Read the model definition and answer for the solid it produces. Units are mm, in the model's axes. Face numbers are marked on the shaded views. A direction names the side the tool comes from. Coordinates: 2 decimals unless noted, no trailing zeros. Write each loop counter-clockwise with the first axis right and the second up, starting at its lowest first coordinate (ties: lowest second). Pieces come first, ordered by that corner, then holes.
from build123d import *

# Parameters (mm, degrees)
BOSS_EXTRUDE1_DEPTH      = 50
BOSS_EXTRUDE1_DEPTH_BACK = 50
SKETCH1_W                = 180
SKETCH1_H                = 152.061
SHELL1_T                 = -5
SKETCH3_W                = 170
SKETCH3_H                = 142.061
BOSS_EXTRUDE2_DEPTH      = 37
CUT_EXTRUDE1_REACH       = 203.694
SKETCH2_W                = 36
SKETCH2_H                = 58
SKETCH4_W                = 36
SKETCH4_H                = 46.5
SKETCH4_R                = 1.5
CUT_EXTRUDE2_DEPTH       = 2
SKETCH4_3_R              = 1.5
CUT_EXTRUDE3_DEPTH       = 132.318836921
SKETCH5_W                = 159.952904784
SKETCH5_H                = 5
CUT_EXTRUDE4_DEPTH       = 63
SKETCH8_W                = 72
SKETCH8_H                = 29.937457508
CUT_EXTRUDE5_DEPTH       = 37
SKETCH9_R                = 1.5
CUT_EXTRUDE6_DEPTH       = 10
CUT_EXTRUDE7_DEPTH       = 102
FILLET1_R                = 10
SKETCH11_W               = 62
SKETCH11_H               = 5
BOSS_EXTRUDE3_DEPTH      = 100
SKETCH12_W               = 57
SKETCH12_H               = 3
SKETCH12_W_2             = 43
SKETCH12_H_2             = 2
CUT_EXTRUDE8_DEPTH       = 91
SKETCH13_W               = 57
SKETCH13_H               = 3
CUT_EXTRUDE9_DEPTH       = 7
FILLET2_R                = 10
FILLET3_R                = 100
SKETCH15_R               = 4
CUT_EXTRUDE10_DEPTH      = 28


with BuildPart() as part:
    # Sketch1 → Boss-Extrude1 (new, two sides: drawn at the far end of the back side and taken through both)
    with BuildSketch(Plane(origin=(0, 0, 0), x_dir=(1, 0, 0), z_dir=(0, 1, 0)).offset(-BOSS_EXTRUDE1_DEPTH_BACK)):
        Rectangle(SKETCH1_W, SKETCH1_H)
    extrude(amount=BOSS_EXTRUDE1_DEPTH + BOSS_EXTRUDE1_DEPTH_BACK)

    # Shell1
    shell1_openings = [part.faces().sort_by_distance(p)[0] for p in [
        (0, -50, 0),
    ]]
    offset(amount=SHELL1_T, openings=shell1_openings, kind=Kind.INTERSECTION)

    # Sketch3 → Boss-Extrude2 (add)
    with BuildSketch(Plane.XZ.offset(-45)):
        Rectangle(SKETCH3_W, SKETCH3_H)
    extrude(amount=BOSS_EXTRUDE2_DEPTH)

    # Sketch2 → Cut-Extrude1 (cut, up to next)
    with BuildSketch(Plane.ZY.offset(90), mode=Mode.PRIVATE) as cut_extrude1_sk1:
        with Locations((-46.0305, -21)):
            Rectangle(SKETCH2_W, SKETCH2_H)
    cut_extrude1_tool1 = extrude(cut_extrude1_sk1.sketch, amount=-CUT_EXTRUDE1_REACH, mode=Mode.PRIVATE) & part.part
    cut_extrude1 = cut_extrude1_tool1.solids().sort_by_distance((-90, -21, -46.0305))[0]
    add(cut_extrude1, mode=Mode.SUBTRACT)

    # Mirror1: Cut-Extrude1 across plane
    add(cut_extrude1.mirror(Plane(origin=(0, 0, 0), x_dir=(0, 0, 1), z_dir=(1, 0, 0))), mode=Mode.SUBTRACT)

    # Sketch4 → Cut-Extrude2 (cut)
    with BuildSketch(Plane.XZ.offset(-8)):
        with Locations((-54, -34.0305)):
            Rectangle(SKETCH4_W, SKETCH4_H)
        with Locations(Location((-43, -50.2805, 0), (0, 0, 270))):
            Circle(SKETCH4_R, mode=Mode.SUBTRACT)
        with Locations(Location((-65, -50.2805, 0), (0, 0, 270))):
            Circle(SKETCH4_R, mode=Mode.SUBTRACT)
        with Locations(Location((-43, -17.7805, 0), (0, 0, 270))):
            Circle(SKETCH4_R, mode=Mode.SUBTRACT)
        with Locations(Location((-65, -17.7805, 0), (0, 0, 270))):
            Circle(SKETCH4_R, mode=Mode.SUBTRACT)
    cut_extrude2 = extrude(amount=-CUT_EXTRUDE2_DEPTH, mode=Mode.SUBTRACT)

    # Sketch4<3> → Cut-Extrude3 (cut, through all)
    with BuildSketch(Plane.XZ.offset(-8)):
        with BuildLine():
            Line((-65, -19.2805), (-65, -17.7805))
            Line((-65, -17.7805), (-63.5, -17.7805))
            ThreePointArc((-63.5, -17.7805), (-66.060660172, -16.719839828), (-65, -19.2805))
        make_face()
        with BuildLine():
            Line((-63.5, -17.7805), (-65, -17.7805))
            Line((-65, -17.7805), (-65, -19.2805))
            ThreePointArc((-65, -19.2805), (-63.939339828, -18.841160172), (-63.5, -17.7805))
        make_face()
        with BuildLine():
            Line((-65, -19.2805), (-65, -17.7805))
            Line((-65, -17.7805), (-63.5, -17.7805))
            ThreePointArc((-63.5, -17.7805), (-66.060660172, -16.719839828), (-65, -19.2805))
        make_face()
        with BuildLine():
            Line((-63.5, -17.7805), (-65, -17.7805))
            Line((-65, -17.7805), (-65, -19.2805))
            ThreePointArc((-65, -19.2805), (-63.939339828, -18.841160172), (-63.5, -17.7805))
        make_face()
        with Locations(Location((-43, -17.7805, 0), (0, 0, 270))):
            Circle(SKETCH4_3_R)
        with Locations(Location((-65, -50.2805, 0), (0, 0, 270))):
            Circle(SKETCH4_3_R)
        with Locations(Location((-43, -50.2805, 0), (0, 0, 270))):
            Circle(SKETCH4_3_R)
    cut_extrude3 = extrude(amount=-CUT_EXTRUDE3_DEPTH, mode=Mode.SUBTRACT)

    # Mirror2: Cut-Extrude2, Cut-Extrude3 across plane
    add(cut_extrude2.mirror(Plane(origin=(0, 0, 0), x_dir=(0, 0, 1), z_dir=(1, 0, 0))), mode=Mode.SUBTRACT)
    add(cut_extrude3.mirror(Plane(origin=(0, 0, 0), x_dir=(0, 0, 1), z_dir=(1, 0, 0))), mode=Mode.SUBTRACT)

    # Sketch5 → Cut-Extrude4 (cut)
    with BuildSketch(Plane.XZ.offset(-8)):
        with Locations((5.023547608, 73.5305)):
            Rectangle(SKETCH5_W, SKETCH5_H)
    extrude(amount=CUT_EXTRUDE4_DEPTH, mode=Mode.SUBTRACT)

    # Sketch8 → Cut-Extrude5 (cut)
    with BuildSketch(Plane.XZ.offset(-8)):
        Polygon((-36, -71.0305), (36, -71.0305), (36, -57.2805), (36, -10.7805), (-36, -10.7805), (-36, -57.2805), align=None)
        with Locations((0, 4.188228754)):
            Rectangle(SKETCH8_W, SKETCH8_H)
        Polygon((36, 19.156957508), (36, -10.7805), (71.419165144, -10.7805), (71.419165144, 76.0305), (-72, 76.0305), (-72, -10.7805), (-36, -10.7805), (-36, 19.156957508), align=None)
    extrude(amount=-CUT_EXTRUDE5_DEPTH, mode=Mode.SUBTRACT)

    # Sketch9 → Cut-Extrude6 (cut)
    with BuildSketch(Plane.XZ.offset(-45)):
        with Locations(Location((31.5, -68.5305, 0), (0, 0, 270))):
            Circle(SKETCH9_R)
        with Locations(Location((-31.5, -68.5305, 0), (0, 0, 270))):
            Circle(SKETCH9_R)
        with Locations(Location((31.5, -8.5305, 0), (0, 0, 270))):
            Circle(SKETCH9_R)
        with Locations(Location((-31.5, -8.5305, 0), (0, 0, 270))):
            Circle(SKETCH9_R)
        with Locations(Location((0, -38.5305, 0), (0, 0, 270))):
            Circle(SKETCH9_R)
    extrude(amount=-CUT_EXTRUDE6_DEPTH, mode=Mode.SUBTRACT)

    # Sketch10 → Cut-Extrude7 (cut)
    with BuildSketch(Plane.XZ.offset(50)):
        Polygon((0, 76.0305), (90, 51.915072681), (90, 76.0305), align=None)
    cut_extrude7 = extrude(amount=-CUT_EXTRUDE7_DEPTH, mode=Mode.SUBTRACT)

    # Mirror3: Cut-Extrude7 across plane
    add(cut_extrude7.mirror(Plane(origin=(0, 0, 0), x_dir=(0, 0, 1), z_dir=(1, 0, 0))), mode=Mode.SUBTRACT)

    # Fillet1
    fillet1_edges = [part.edges().sort_by_distance(p)[0] for p in [
        (0, 47.5, 76.0305),
    ]]
    fillet(fillet1_edges, radius=FILLET1_R)

    # Sketch11 → Boss-Extrude3 (add)
    with BuildSketch(Plane.XZ.offset(50)):
        Polygon((85, -86.0305), (85, -76.0305), (-85, -76.0305), (-85, -86.0305), (-31, -86.0305), (31, -86.0305), align=None)
        with Locations((0, -88.5305)):
            Rectangle(SKETCH11_W, SKETCH11_H)
    extrude(amount=-BOSS_EXTRUDE3_DEPTH)

    # Sketch12 → Cut-Extrude8 (cut)
    with BuildSketch(Plane.XZ.offset(50)):
        with Locations((0, -87.5305)):
            Rectangle(SKETCH12_W, SKETCH12_H)
        with Locations((0, -90.0305)):
            Rectangle(SKETCH12_W_2, SKETCH12_H_2)
    extrude(amount=-CUT_EXTRUDE8_DEPTH, mode=Mode.SUBTRACT)

    # Sketch13 → Cut-Extrude9 (cut)
    with BuildSketch(Plane.XZ.offset(-41)):
        with Locations((0, -87.5305)):
            Rectangle(SKETCH13_W, SKETCH13_H)
    extrude(amount=-CUT_EXTRUDE9_DEPTH, mode=Mode.SUBTRACT)

    # Fillet2
    # the kernel refuses this fillet: 10 mm, written as the material it takes off along each edge
    with BuildSketch(Plane(origin=(90, -71.650635095, -76.0305), x_dir=(0, 0, 1), z_dir=(0, 1, 0))) as fillet2_piece_1:
        with BuildLine():
            CenterArc((8.660254038, -10), FILLET2_R, 90, 60)
            Line((0, -5), (-0.173205081, -4.9))
            ThreePointArc((-0.173205081, -4.9), (-0.2, -2.5), (-0.2, 0))
            Line((-0.2, 0), (0, 0.2))
            Line((0, 0.2), (8.660254038, 0.2))
            Line((8.660254038, 0.2), (8.660254038, 0))
        make_face()
    extrude(amount=143.301270189, mode=Mode.SUBTRACT)
    with BuildSketch(Plane(origin=(-90, 71.650635095, -76.0305), x_dir=(1, 0, 0), z_dir=(0, -1, 0))) as fillet2_piece_2:
        with BuildLine():
            CenterArc((10, 8.660254038), FILLET2_R, 180, 60)
            Line((0, 8.660254038), (-0.2, 8.660254038))
            Line((-0.2, 8.660254038), (-0.2, 0))
            Line((-0.2, 0), (0, -0.2))
            ThreePointArc((0, -0.2), (2.5, -0.2), (4.9, -0.173205081))
            Line((4.9, -0.173205081), (5, 0))
        make_face()
    extrude(amount=143.301270189, mode=Mode.SUBTRACT)

    # Fillet3
    # the kernel refuses this fillet: 100 mm, written as the material it takes off along each edge
    with BuildSketch(Plane(origin=(-85, -158.972473589, -86.0305), x_dir=(1, 0, 0), z_dir=(0, 1, 0))) as fillet3_piece_1:
        with BuildLine():
            CenterArc((43.588989435, -100), FILLET3_R, 90, 25.841932763)
            Line((0, -10), (0, 0))
            Line((0, 0), (43.588989435, 0))
        make_face()
    extrude(amount=317.944947177, mode=Mode.SUBTRACT)
    with BuildSketch(Plane(origin=(85, -158.972473589, -86.0305), x_dir=(0, 0, 1), z_dir=(0, 1, 0))) as fillet3_piece_2:
        with BuildLine():
            CenterArc((100, -43.588989435), FILLET3_R, 154.158067237, 25.841932763)
            Line((0, -43.588989435), (0, 0))
            Line((0, 0), (10, 0))
        make_face()
    extrude(amount=317.944947177, mode=Mode.SUBTRACT)

    # Sketch15 → Cut-Extrude10 (cut)
    with BuildSketch(Plane(origin=(0, 50, 0), x_dir=(1, 0, 0), z_dir=(0, 1, 0))):
        with Locations(Location((65, 17.7805, 0), (0, 0, 270))):
            Circle(SKETCH15_R)
        with Locations(Location((43, 17.7805, 0), (0, 0, 270))):
            Circle(SKETCH15_R)
        with Locations(Location((65, 50.2805, 0), (0, 0, 270))):
            Circle(SKETCH15_R)
        with Locations(Location((-43, 50.2805, 0), (0, 0, 90))):
            Circle(SKETCH15_R)
        with Locations(Location((43, 50.2805, 0), (0, 0, 270))):
            Circle(SKETCH15_R)
        with Locations(Location((-65, 50.2805, 0), (0, 0, 90))):
            Circle(SKETCH15_R)
        with Locations(Location((-43, 17.7805, 0), (0, 0, 90))):
            Circle(SKETCH15_R)
        with Locations(Location((-65, 17.7805, 0), (0, 0, 90))):
            Circle(SKETCH15_R)
    extrude(amount=-CUT_EXTRUDE10_DEPTH, mode=Mode.SUBTRACT)


solid = part.part
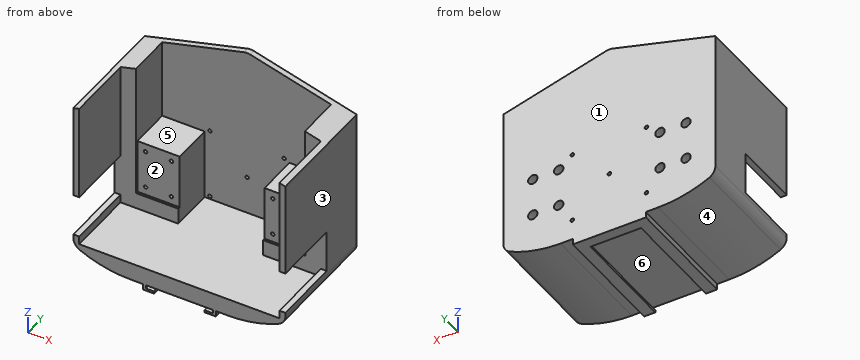
Item 1: The part is cut by section A-A (y = -1.5). State how many separate pieces and enclosed holes the cut face has, and give its area (3 significant figures).
Item 2: Determine the mould class of the marked faces 1, 2 and 3 for opening direction X: +X half, -X half, draft (parallel to the pull), parting line (faces both ways), or undercut.
Item 3: Find the intervals of material crossed by probe 1 along X at (y, z) = (37, -59.5); probe 2 along X at (y, z) = (-33, -11.5); probe 3 along Z at (x, y) = (-43.5, 46.5), in increasing order.
Item 4: Given pin 1 (1.5 mm diameter, centred on x = 54, y = -0.5, fed in from +Z); pin 2 (8.5 mm diameter, centred on x = 35.5, y = 16.5, fed in from -Z); pin 3 (6 mm diameter, centred on x = 7.5, z = 9.5, fed in from -Y); pin 4 (6.5 mm diameter, centred on x = -42, z = -49.5, fed in from +Y), each flat-ended and moving along its own axis, determine where each tip first touches the part or whether it passes through.
Item 5: For the marked faces 4, 5 and 6, determine the directions among +Z, -Z, +X, -X, +Y, -Y from which every point of the face is accessible in a straight line to the end or side of a thin tool.
Item 6: The part is cut by section B-B (z = 42). Give the vertices of the cut face in (x, y).
Answer:
1. separate pieces: 3
1. enclosed holes: 0
1. area: 3,220 mm2
2. face 1: draft
2. face 2: undercut
2. face 3: +X half
3. probe 1: x = -90 to -36, 36 to 90
3. probe 2: x = -90 to -85, 85 to 90
3. probe 3: z = -86.01 to -54.25, -46.31 to -21.75, -13.81 to 64.37
4. pin 1: stops at z = -71.03
4. pin 2: stops at z = -86.03
4. pin 3: stops at y = 45
4. pin 4: stops at y = 50
5. face 4: -Z, -X, +Y, -Y
5. face 5: +Z, -Y
5. face 6: -Y
6. outline: (-90, -50) - (-85, -50) - (-85, 8) - (-72, 8) - (-72, 45) - (71.42, 45) - (71.42, 8) - (85, 8) - (85, -50) - (90, -50) - (90, 50) - (-90, 50) - close
